```python
from build123d import *

# Parameters (mm, degrees)
SKETCH001_R   = 26
EXTRUDE_DEPTH = 10
BOX_W         = 100
BOX_H         = 100
BOX_DEPTH     = 4


with BuildPart() as glass_holder_hole:
    # Sketch001 (on Face5 of Box) → Extrude (new body)
    with BuildSketch(Plane(origin=(-50, -50, 0), x_dir=(1, 0, 0), z_dir=(0, 0, -1))):
        with Locations((50, -50)):
            Circle(SKETCH001_R)
    extrude(amount=-EXTRUDE_DEPTH)


with BuildPart() as glass_holder:
    # Box → Box (new body)
    with BuildSketch(Plane(origin=(-50, -50, 0), x_dir=(1, 0, 0), z_dir=(0, 0, 1))):
        with Locations((50, 50)):
            Rectangle(BOX_W, BOX_H)
    extrude(amount=BOX_DEPTH)

    # Cut: cut Glass Holder Hole
    add(glass_holder_hole.part, mode=Mode.SUBTRACT)


solid = glass_holder.part
```
Work out the finished part from the listing and answer in its coordinate system (mm). Give positions to 0.01 mm unless a question says otherwise; leave off trailing zeros. Write each loop counter-clockwise with the first axis right and the second up, starting at its lowest first coordinate (ties: lowest second). Pieces come first, ordered by that corner, then holes.
(1) The part is cut by section A-A on x = 0. Write down the section's boundary in (y, z), plus the area to 3 significant figures.
Final values:
outline: (-50, 0) - (-26, 0) - (-26, 4) - (-50, 4) - close; (26, 0) - (50, 0) - (50, 4) - (26, 4) - close
area: 192 mm2
(2) The mould has two halves that part along Y. Classify faces 1 (the flat face through (-23, 23, 0)), 2 (the flat face through (-1, -50, 2)), 3 (the cylindrical face through (-20.633, 15.821, 1.972)), 4 (the flat face through (-1, 50, 2)): pulls with the +Y half, pulls with the -Y half, needs draft (parallel to the pull), parting line crosses it, or undercut.
Final values:
face 1: needs draft
face 2: pulls with the -Y half
face 3: undercut
face 4: pulls with the +Y half
(3) The part is cut by section C-C on z = 1.25. Write down the section's boundary in (x, y).
Final values:
outline: (-50, -50) - (50, -50) - (50, 50) - (-50, 50) - close; hole circle Ø52 at (0, 0)
(4) Straight lines are drawn through the part: line 1 (X direction, y = 0, z = 2.65); line 2 (Y direction, x = -17.5, z = 1.5). For each, find the intervals that lie inside material, in ascending order.
Final values:
line 1: x = -50 to -26, 26 to 50
line 2: y = -50 to -19.23, 19.23 to 50
